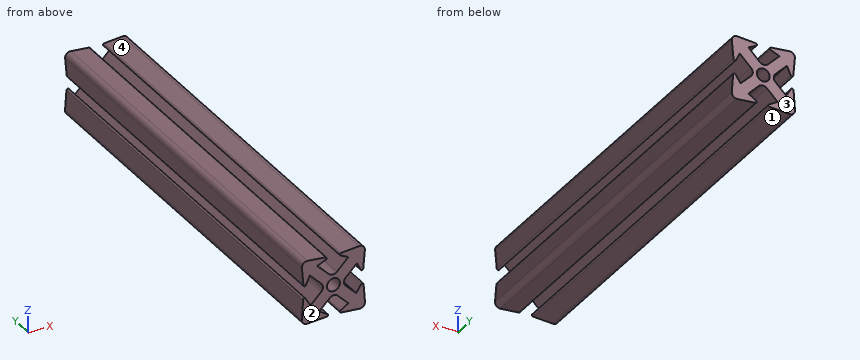
```python
from build123d import *

# Parameters (mm, degrees)
BOSS_EXTRUDE1_DEPTH     = 603.25
SKETCH8_R               = 2.565266714
CUT_EXTRUDE4_DEPTH      = 604.996
FILLET1_R               = 2.032
FILLET2_R               = 0.508
SKETCH5_W               = 12.655737404
SKETCH5_H               = 275.477439744
BOSS_EXTRUDE3_DEPTH     = 4.572
SKETCH6_R               = 4.617709461
SKETCH6_R_2             = 4.503643825
SKETCH6_R_3             = 4.621904919
SKETCH6_R_4             = 4.672748293
SKETCH6_R_5             = 4.615964847
CUT_EXTRUDE2_DEPTH      = 4.572
SKETCH7_R               = 4.54487388
SKETCH7_R_2             = 4.672668652
CUT_EXTRUDE3_DEPTH      = 4.572
FILLET3_R               = 2.286
CUT_EXTRUDE6_DEPTH      = 10.922
CUT_EXTRUDE6_DEPTH_BACK = 38.354
SKETCH9_W               = 60.400846089
SKETCH9_H               = 376.70446786
CUT_EXTRUDE7_DEPTH      = 11.938
CUT_EXTRUDE7_DEPTH_BACK = 33.274
SKETCH10_W              = 57.705662998
SKETCH10_H              = 86.678631682


with BuildPart() as part:
    # Sketch2 → Boss-Extrude1 (new body)
    with BuildSketch(Plane(origin=(0, 0, 0), x_dir=(1, 0, 0), z_dir=(0, 1, 0))):
        Polygon((-16.258611825, -14.593573265), (-15.211300169, -2.97584616), (-12.901409331, -8.316313776), (2.370242199, 7.164742979), (-1.981461576, 9.939777323), (9.141388175, 10.806426735), (8.274738763, -0.316423015), (5.499704418, 4.03528076), (-9.981352337, -11.236370771), (-4.640884721, -13.546261608), align=None)
        Polygon((-15.391962413, -0.962649654), (-12.616928069, 3.750799497), (2.370242199, -11.236370771), (-2.346798037, -13.546261608), (9.141388175, -14.593573265), (8.094076519, -3.105387053), (5.784185681, -7.822427289), (-9.202984587, 7.164742979), (-4.489535436, 9.939777323), (-16.258611825, 10.806426735), align=None)
    extrude(amount=BOSS_EXTRUDE1_DEPTH)

    # Sketch8 → Cut-Extrude4 (cut)
    with BuildSketch(Plane(origin=(0, 603.25, 0), x_dir=(1, 0, 0), z_dir=(0, 1, 0))):
        with Locations(Location((-3.527048706, -1.915222876, 0), (0, 0, 270))):
            Circle(SKETCH8_R)
    extrude(amount=-CUT_EXTRUDE4_DEPTH, mode=Mode.SUBTRACT)

    # Fillet1
    fillet1_edges = [part.edges().sort_by_distance(p)[0] for p in [
        (9.141388175, 301.625, -10.806426735),
        (9.141388175, 301.625, 14.593573265),
        (-16.258611825, 301.625, 14.593573265),
        (-16.258611825, 301.625, -10.806426735),
    ]]
    fillet(fillet1_edges, radius=FILLET1_R)

    # Fillet2
    fillet2_edges = [part.edges().sort_by_distance(p)[0] for p in [
        (-1.981461576, 301.625, -9.939777323),
        (8.274738763, 301.625, 0.316423015),
        (8.094076519, 301.625, 3.105387053),
        (-2.346798037, 301.625, 13.546261608),
        (-4.640884721, 301.625, 13.546261608),
        (-15.211300169, 301.625, 2.97584616),
        (-15.391962413, 301.625, 0.962649654),
        (-4.489535436, 301.625, -9.939777323),
    ]]
    fillet(fillet2_edges, radius=FILLET2_R)

    # Sketch5 → Boss-Extrude3 (add)
    with BuildSketch(Plane(origin=(-0.781752329, 0, -10.033254025), x_dir=(-0.9969782897972478, 0, 0.07768069047681715), z_dir=(-0.07768069047681715, 0, -0.9969782897972478))):
        with Locations((2.46042797, 432.716085527)):
            Rectangle(SKETCH5_W, SKETCH5_H)
    extrude(amount=BOSS_EXTRUDE3_DEPTH)

    # Sketch6 → Cut-Extrude2 (cut)
    with BuildSketch(Plane(origin=(-1.136908446, 0, -14.591438766), x_dir=(-0.9969782897972478, 0, 0.07768069047681722), z_dir=(-0.07768069047681722, 0, -0.9969782897972478))):
        with Locations((2.46042797, 545.232588529)):
            Circle(SKETCH6_R)
        with Locations((2.46042797, 513.854170907)):
            Circle(SKETCH6_R_2)
        with Locations((2.46042797, 479.255100803)):
            Circle(SKETCH6_R_3)
        with Locations((2.46042797, 446.301604006)):
            Circle(SKETCH6_R_4)
        with Locations((2.46042797, 414.342225806)):
            Circle(SKETCH6_R_5)
    extrude(amount=-CUT_EXTRUDE2_DEPTH, mode=Mode.SUBTRACT)

    # Sketch7 → Cut-Extrude3 (cut)
    with BuildSketch(Plane(origin=(-1.136908446, 0, -14.591438766), x_dir=(-0.9969782897972478, 0, 0.07768069047681712), z_dir=(-0.07768069047681712, 0, -0.9969782897972478))):
        with Locations((2.610241648, 377.377881706)):
            Circle(SKETCH7_R)
        with Locations((2.157369038, 338.135767483)):
            Circle(SKETCH7_R_2)
    extrude(amount=-CUT_EXTRUDE3_DEPTH, mode=Mode.SUBTRACT)

    # Fillet3
    fillet3_edges = [part.edges().sort_by_distance(p)[0] for p in [
        (-0.326311914, 301.625, 1.711929695),
        (-6.767665082, 301.625, 2.09846349),
        (-3.376968255, 301.625, -1.338726647),
        (-3.76350205, 301.625, 5.102626521),
    ]]
    fillet(fillet3_edges, radius=FILLET3_R)

    # Sketch9 → Cut-Extrude6 (cut, two sides: drawn at the far end of the back side and taken through both)
    with BuildSketch(Plane(origin=(-14.822577076, 0, -1.336221587), x_dir=(-0.08978364374222932, 0, 0.995961293081397), z_dir=(-0.9959612930813971, 0, -0.08978364374222933)).offset(-CUT_EXTRUDE6_DEPTH_BACK)):
        with Locations((4.674775329, 432.715581258)):
            Rectangle(SKETCH9_W, SKETCH9_H)
    extrude(amount=CUT_EXTRUDE6_DEPTH + CUT_EXTRUDE6_DEPTH_BACK, mode=Mode.SUBTRACT)

    # Sketch10 → Cut-Extrude7 (cut, two sides: drawn at the far end of the back side and taken through both)
    with BuildSketch(Plane(origin=(7.74659499, 0, -0.706212372), x_dir=(-0.09078774644161682, 0, -0.9958702651932394), z_dir=(0.9958702651932394, 0, -0.09078774644161682)).offset(-CUT_EXTRUDE7_DEPTH_BACK)):
        with Locations((-4.603685072, 208.51404869)):
            Rectangle(SKETCH10_W, SKETCH10_H)
    extrude(amount=CUT_EXTRUDE7_DEPTH + CUT_EXTRUDE7_DEPTH_BACK, mode=Mode.SUBTRACT)


solid = part.part
```
The listing builds one solid part. Answer for the finished solid, in the listing's coordinates (mm). Face numbers are marked on the shaded views. A direction names the side the tool comes from. Coordinates: 2 decimals unless noted, no trailing zeros. Write item = value, one per line.
1) Find the intervals of material crossed by line 1 along X through (y, z) = (27, -1.25); line 2 along X through (y, z) = (20, -1.75); line 3 along X through (y, z) = (83, 0.5), in increasing order.
Responses:
line_1 = -15.55 to -14.09, -10.12 to 2.68, 7.28 to 8.4
line_2 = -15.59 to -13.79, -10.62 to 3.18, 6.96 to 8.44
line_3 = -8.37 to -5.67, -1.39 to 0.99
2) Which of the six approach directions +Z, -Z, +X, -X, +Y, -Y give full straight-line access (tool end or side, diameter ignored) to the marked faces 3 and 4?
Responses:
face_3 = +Z, -Z, +X, -X, +Y
face_4 = +Z, +Y, -Y
3) Determine the mould class of the marked faces 1 and 2 for opening direction X: pulls with the +X half, pulls with the -X half, needs draft (parallel to the pull), parting line crosses it, or undercut.
Responses:
face_1 = undercut
face_2 = needs draft
4) Each of these flat-tipped pins is pushed along its axis until it touches: P1, Ø3, axis at x = -3.53, z = 1.92, coming from the +Y side; P2, Ø1, axis at y = 33.5, z = 0, coming from the -X side; P3, Ø6, axis at x = -4.5, y = 51, coming from the -Z side; P4, Ø10, axis at x = -8.5, y = 147.5, coming from the -Z side. Where does it stop, or does it pass through?
Responses:
P1 = through
P2 = -15.47
P3 = -10.16
P4 = -10.6
